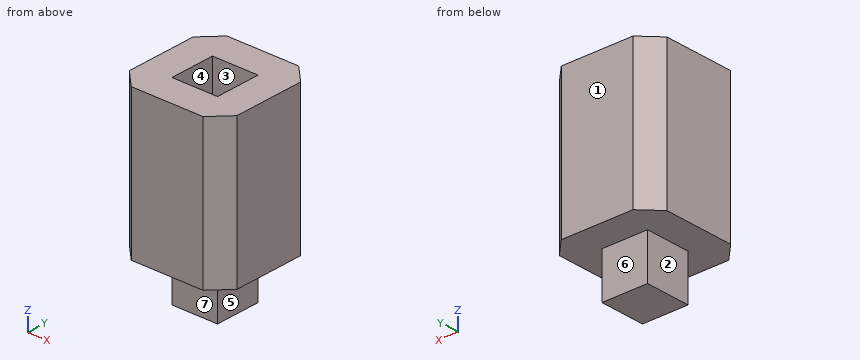
from build123d import *

# Parameters (mm, degrees)
F0_W     = 60
F0_H     = 60
F1_DEPTH = 82
F2_SIZE  = 10
F3_W     = 25.4
F3_H     = 25.4
F4_DEPTH = 25.4
F5_W     = 25.4
F5_H     = 25.4
F6_DEPTH = 25.4


with BuildPart() as f1:
    # F0 (on Top) → F1 (new body)
    with BuildSketch(Plane.XY):
        Rectangle(F0_W, F0_H)
    extrude(amount=F1_DEPTH)

    # F2
    f2_edges = [f1.edges().sort_by_distance(p)[0] for p in [
        (30, -30, 41),
        (30, 30, 41),
        (-30, -30, 41),
        (-30, 30, 41),
    ]]
    chamfer(f2_edges, length=F2_SIZE)

    # F3 (on face) → F4 (cut)
    with BuildSketch(Plane.XY.offset(82)):
        Rectangle(F3_W, F3_H)
    extrude(amount=-F4_DEPTH, mode=Mode.SUBTRACT)

    # F5 (on face) → F6 (join)
    with BuildSketch(Plane(origin=(0, 0, 0), x_dir=(1, 0, 0), z_dir=(0, 0, -1))):
        Rectangle(F5_W, F5_H)
    extrude(amount=F6_DEPTH)


solid = f1.part
Work out the finished part from the listing and answer in its coordinate system (mm). Face numbers are marked on the shaded views. A direction names the side the tool comes from. Give positions to 0.01 mm unless a question says otherwise; leave off trailing zeros. Loops run counter-clockwise (first coordinate to the right, second up) from the corner with the lowest first, then second, coordinate; pieces in that order, holes last. Notation, with made-up numbers: (82.5, -26) - (92.5, -26) arc R29 ccw to (92.5, 3) - close; hole circle Ø8 at (-30, 51). An arc over 180 degrees is marked (long way). Answer in a Markdown table with one row per item. Add a question column.
Q1. Consider line 1 along X through (y, z) = (-5.5, 69); line 2 along Z through (x, y) = (21, -21). Determine where each line is inside the solid, lowest interval first.
Q2. A tool of negligible diameter and unlimited length cuts with its end or side. For the marked faces 4, 5, 6 and 7, from which of +Z, -Z, +X, -X, +Y, -Y can it reach the whole face along a straight path? Write none if from no direction.
Q3. The part is cut by section D-D (y = -24). Determine the outline of the cut face in (x, z).
Q4. Each of these flat-tipped pins is pushed along its axis until it touches: P1, Ø12.5, axis at x = 3.5, y = -2.5, coming from the +Z side; P2, Ø20.5, axis at x = 1, z = -13, coming from the +Y side; P3, Ø4, axis at x = 15.5, y = 6, coming from the -Z side. Where does it stop, or does it pass through?
Q5. The part is cut by section B-B (x = -6). Determine the outline of the cut face in (y, z), and give its area (3 significant figures).
Q6. Determine the mould class of the marked faces 1, 2 and 3 for opening direction Y: released by +Y, released by -Y, zero draft, split by the parting line, or undercut.
Q7. The part is cut by section A-A (z = 22). Determine the outline of the cut face in (x, y), and give its area (3 significant figures).
Solution:
| question | item | result |
|---|---|---|
| 1 | line 1 | x = -30 to -12.7, 12.7 to 30 |
| 1 | line 2 | z = 0 to 82 |
| 2 | face 4 | +Z |
| 2 | face 5 | -Z, +X, +Y, -Y |
| 2 | face 6 | -Z, +X, -X, +Y |
| 2 | face 7 | -Z, +X, -X, -Y |
| 3 | outline | (-26, 0) - (26, 0) - (26, 82) - (-26, 82) - close |
| 4 | P1 | stops at z = 56.6 |
| 4 | P2 | stops at y = 12.7 |
| 4 | P3 | stops at z = 0 |
| 5 | outline | (-30, 0) - (-12.7, 0) - (-12.7, -25.4) - (12.7, -25.4) - (12.7, 0) - (30, 0) - (30, 82) - (12.7, 82) - (12.7, 56.6) - (-12.7, 56.6) - (-12.7, 82) - (-30, 82) - close |
| 5 | area | 4,920 mm² |
| 6 | face 1 | released by +Y |
| 6 | face 2 | zero draft |
| 6 | face 3 | undercut |
| 7 | outline | (-30, -20) - (-20, -30) - (20, -30) - (30, -20) - (30, 20) - (20, 30) - (-20, 30) - (-30, 20) - close |
| 7 | area | 3,400 mm² |
